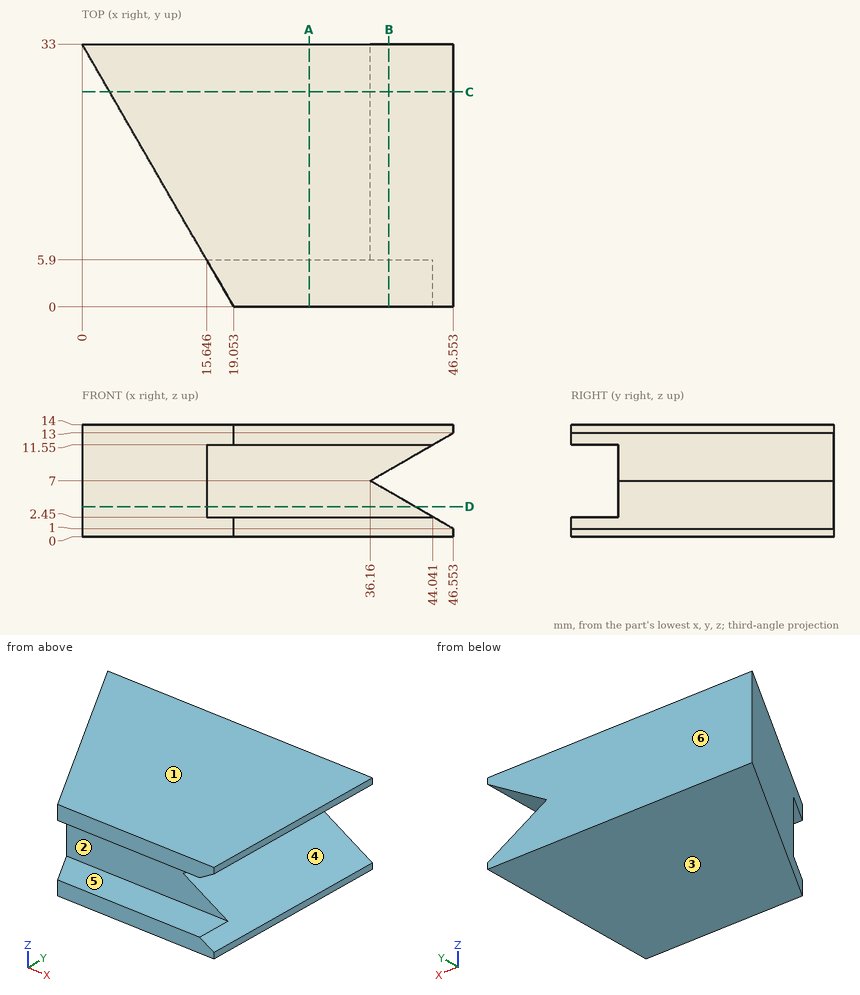
Geometry: see drawing. Coordinates: mm, zero at the bounding-box minimum. A direction names the side the tool comes from. Round coordinates to 2 decimals unless told otherwise and drop trailing zeros. Loops run counter-clockwise (first coordinate to the right, second up) from the corner with the lowest first, then second, coordinate; pieces in that order, holes last. Notation, with made-up numbers: (69.5, 17.25) -> (84.5, 17.25) arc R22 cw to (84.5, 30.25) -> close; hole circle Ø1 at (85, 15.25). An arc over 180 degrees is marked (long way). Write each question's results on one line, items separated by ' | '.
1. Ray query, line 1 (Z direction, x = 22, y = 3.5); line 2 (Y direction, x = 31.5, z = 10.75); line 3 (Z direction, x = 42.5, y = 18.5). Return the intervals inside material, ascending. Write a range as from..to.
Geometry results:
line 1: 0..2.45, 11.55..14 | line 2: 5.9..33 | line 3: 0..3.34, 10.66..14
2. Section A-A (x = 28.5). Return loops of the section in (y, z), and give its area (3 significant figures).
Geometry results:
outline: (0, 0) -> (33, 0) -> (33, 14) -> (0, 14) -> (0, 11.55) -> (5.9, 11.55) -> (5.9, 2.45) -> (0, 2.45) -> close | area: 408 mm2
3. First-contact query: P1, Ø6, axis at y = 11.5, z = 8, coming from the -X side; P2, Ø2.5, axis at x = 33.5, z = 7, coming from the -Y side. Flat tips, straight axial feed; report the tip coordinate or a pass-through.
Geometry results:
P1: x = 10.68 | P2: y = 5.9
4. Section C-C (y = 27). Return loops of the section in (x, z).
Geometry results:
outline: (3.46, 0) -> (46.55, 0) -> (46.55, 1) -> (36.16, 7) -> (46.55, 13) -> (46.55, 14) -> (3.46, 14) -> close
5. Section B-B (x = 38.5). Return loops of the section in (y, z), and give its area (3 significant figures).
Geometry results:
outline: (0, 0) -> (33, 0) -> (33, 5.65) -> (5.9, 5.65) -> (5.9, 2.45) -> (0, 2.45) -> close; (0, 11.55) -> (5.9, 11.55) -> (5.9, 8.35) -> (33, 8.35) -> (33, 14) -> (0, 14) -> close | area: 335 mm2
6. Section D-D (z = 3.75). Return loops of the section in (x, y).
Geometry results:
outline: (0, 33) -> (15.65, 5.9) -> (41.79, 5.9) -> (41.79, 33) -> close
7. Mould query, pull axis Z, two halves, no side actions, for the marked faces 3, 4, 5 and 6. Classes: +Z half, -Z half, draft (parallel to the pull), parting line (faces both ways), or undercut.
Geometry results:
face 3: -Z half | face 4: undercut | face 5: undercut | face 6: draft
8. Set-up query: the marked faces 1 and 2. Return all of +Z, -Z, +X, -X, +Y, -Y with unobstructed straight access to the full face (end or side cutting, diameter ignored); none if empty.
Geometry results:
face 1: +Z, +X, -X, +Y, -Y | face 2: +X, -X, -Y
